Can you work these out from the model? Positions are in its coordinate system, mm. A direction names the side the tool comes from. Coordinates: 2 decimals unless noted, no trailing zeros. Order: outer loops, then holes, each group sorted by start corner. A loop starts at its lowest first (then second) coordinate and runs counter-clockwise, first axis right, second up.
```python
from build123d import *

# Parameters (mm, degrees)
EXTRUDE_1_DEPTH     = 10
SKETCH_2_R          = 1.25
CUT_EXTRUDE_1_DEPTH = 15
SKETCH_4_R          = 0.95
CUT_EXTRUDE_2_DEPTH = 40.749213829
EXTRUDE_2_DEPTH     = 28
SKETCH_7_W          = 6
SKETCH_7_H          = 20
EXTRUDE_4_DEPTH     = 2
CHAMFER_1_SIZE      = 0.6
EXTRUDE_5_DEPTH     = 10
FILLET_2_R          = 6
CUT_EXTRUDE_3_DEPTH = 1
CHAMFER_2_SIZE      = 1


# Some blends are built 0.0001 mm under size
with BuildPart() as part:
    # 草图1 → 凸台-拉伸1 (new, symmetric)
    with BuildSketch(Plane(origin=(0, 0, 0), x_dir=(1, 0, 0), z_dir=(0, 1, 0))):
        Polygon((0, 0), (3, 0), (3, 10), (1, 10), (1, 2), (-2, 2), (-2, -26), (-6, -26), (-6, -28), (0, -28), align=None)
    extrude(amount=EXTRUDE_1_DEPTH, both=True)

    # 草图2 → 切除-拉伸1 (cut)
    with BuildSketch(Plane.ZY.offset(-1)):
        with Locations((-5, 0)):
            Circle(SKETCH_2_R)
    extrude(amount=-CUT_EXTRUDE_1_DEPTH, mode=Mode.SUBTRACT)

    # 草图4 → 切除-拉伸2 (cut, through all)
    with BuildSketch(Plane.XY.offset(28)):
        with Locations((-4, 0)):
            Circle(SKETCH_4_R)
    extrude(amount=-CUT_EXTRUDE_2_DEPTH, mode=Mode.SUBTRACT)

    # 草图5 → 凸台-拉伸2 (add)
    with BuildSketch(Plane(origin=(0, 0, 26), x_dir=(-1, 0, 0), z_dir=(0, 0, -1))):
        Polygon((2, 10), (6, 10), (2, 6), align=None)
        Polygon((2, -6), (2, -10), (6, -10), align=None)
    extrude(amount=EXTRUDE_2_DEPTH)

    # 草图7 → 凸台-拉伸4 (add)
    with BuildSketch(Plane(origin=(0, 0, -10), x_dir=(-1, 0, 0), z_dir=(0, 0, -1))):
        with Locations((-4, 0)):
            Rectangle(SKETCH_7_W, SKETCH_7_H)
    extrude(amount=EXTRUDE_4_DEPTH)

    # 倒角1
    chamfer_1_edges = [part.edges().sort_by_distance(p)[0] for p in [
        (5, 10, -10),
        (5, -10, -10),
    ]]
    chamfer(chamfer_1_edges, length=CHAMFER_1_SIZE)

    # 草图8 → 凸台-拉伸5 (add)
    with BuildSketch(Plane(origin=(0, 0, -2), x_dir=(-1, 0, 0), z_dir=(0, 0, -1))):
        Polygon((-1, 10), (1.5, 10), (-1, 7.5), align=None)
        Polygon((-1, -7.5), (-1, -10), (1.5, -10), align=None)
    extrude(amount=EXTRUDE_5_DEPTH)

    # 圆角2
    # the kernel refuses this fillet: 6 mm, written as the material it adds along each edge
    with BuildSketch(Plane(origin=(-12.106601718, -20.606601718, -2), x_dir=(-0.7071067811865437, 0.7071067811865513, 0), z_dir=(0.7071067811865513, 0.7071067811865438, 0))) as fillet_2_piece_1_section:
        with BuildLine():
            CenterArc((FILLET_2_R, -FILLET_2_R), FILLET_2_R, 90, 90)
            Line((0, -FILLET_2_R), (0, 0))
            Line((0, 0), (FILLET_2_R, 0))
        make_face()
    fillet_2_piece_1 = extrude(amount=33.535533906, mode=Mode.PRIVATE)
    fillet_2_piece_1 = split(fillet_2_piece_1, bisect_by=Plane(origin=(-2, -8.855149606, -2.774001208), z_dir=(-1, 0, 0)), keep=Keep.TOP, mode=Mode.PRIVATE)
    fillet_2_piece_1 = split(fillet_2_piece_1, bisect_by=Plane(origin=(-4, -8, -2.774001208), z_dir=(0.7071067811865515, -0.7071067811865436, 0)), keep=Keep.TOP, mode=Mode.PRIVATE)
    fillet_2_piece_1 = split(fillet_2_piece_1, bisect_by=Plane(origin=(-3.144850394, -10, -2.774001208), z_dir=(0, 1, 0)), keep=Keep.TOP, mode=Mode.PRIVATE)
    add(fillet_2_piece_1)
    with BuildSketch(Plane(origin=(-12.106601718, -20.606601718, -2), x_dir=(-0.7071067811865437, 0.7071067811865513, 0), z_dir=(0.7071067811865513, 0.7071067811865438, 0))) as fillet_2_piece_2_section:
        with BuildLine():
            CenterArc((FILLET_2_R, -FILLET_2_R), FILLET_2_R, 90, 90)
            Line((0, -FILLET_2_R), (0, 0))
            Line((0, 0), (FILLET_2_R, 0))
        make_face()
    fillet_2_piece_2 = extrude(amount=33.535533906, mode=Mode.PRIVATE)
    fillet_2_piece_2 = split(fillet_2_piece_2, bisect_by=Plane(origin=(1, -3.168547951, -2.116110368), z_dir=(-1, 0, 0)), keep=Keep.TOP, mode=Mode.PRIVATE)
    fillet_2_piece_2 = split(fillet_2_piece_2, bisect_by=Plane(origin=(-2, -3.168547951, -2.116110368), z_dir=(1, 0, 0)), keep=Keep.TOP, mode=Mode.PRIVATE)
    fillet_2_piece_2 = split(fillet_2_piece_2, bisect_by=Plane(origin=(0.165726024, -3.834273976, -2.116110368), z_dir=(-0.7071067811865515, 0.7071067811865436, 0)), keep=Keep.TOP, mode=Mode.PRIVATE)
    add(fillet_2_piece_2)
    with BuildSketch(Plane(origin=(-12.106601718, -20.606601718, -2), x_dir=(-0.7071067811865437, 0.7071067811865513, 0), z_dir=(0.7071067811865513, 0.7071067811865438, 0))) as fillet_2_piece_3_section:
        with BuildLine():
            CenterArc((FILLET_2_R, -FILLET_2_R), FILLET_2_R, 90, 90)
            Line((0, -FILLET_2_R), (0, 0))
            Line((0, 0), (FILLET_2_R, 0))
        make_face()
    fillet_2_piece_3 = extrude(amount=33.535533906, mode=Mode.PRIVATE)
    fillet_2_piece_3 = split(fillet_2_piece_3, bisect_by=Plane(origin=(1, -7.448559775, -3.464262476), z_dir=(-1, 0, 0)), keep=Keep.TOP, mode=Mode.PRIVATE)
    fillet_2_piece_3 = split(fillet_2_piece_3, bisect_by=Plane(origin=(-2, -7.448559775, -3.464262476), z_dir=(1, 0, 0)), keep=Keep.TOP, mode=Mode.PRIVATE)
    fillet_2_piece_3 = split(fillet_2_piece_3, bisect_by=Plane(origin=(-1.950921276, -5.950921276, -3.464262476), z_dir=(0.7071067811865515, -0.7071067811865436, 0)), keep=Keep.TOP, mode=Mode.PRIVATE)
    fillet_2_piece_3 = split(fillet_2_piece_3, bisect_by=Plane(origin=(-0.453282777, -10, -3.464262476), z_dir=(0, 1, 0)), keep=Keep.TOP, mode=Mode.PRIVATE)
    add(fillet_2_piece_3)
    with BuildSketch(Plane(origin=(-12.106601718, 20.606601718, -2), x_dir=(-0.707106781186544, -0.7071067811865511, 0), z_dir=(0.7071067811865511, -0.7071067811865439, 0))) as fillet_2_piece_4_section:
        with BuildLine():
            CenterArc((FILLET_2_R, FILLET_2_R), FILLET_2_R, 180, 90)
            Line((0, FILLET_2_R), (0, 0))
            Line((0, 0), (FILLET_2_R, 0))
        make_face()
    fillet_2_piece_4 = extrude(amount=33.535533906, mode=Mode.PRIVATE)
    fillet_2_piece_4 = split(fillet_2_piece_4, bisect_by=Plane(origin=(-3.144850394, 10, -2.774001208), z_dir=(0, -1, 0)), keep=Keep.TOP, mode=Mode.PRIVATE)
    fillet_2_piece_4 = split(fillet_2_piece_4, bisect_by=Plane(origin=(-4, 8, -2.774001208), z_dir=(0.7071067811865515, 0.7071067811865436, 0)), keep=Keep.TOP, mode=Mode.PRIVATE)
    fillet_2_piece_4 = split(fillet_2_piece_4, bisect_by=Plane(origin=(-2, 8.855149606, -2.774001208), z_dir=(-1, 0, 0)), keep=Keep.TOP, mode=Mode.PRIVATE)
    add(fillet_2_piece_4)
    with BuildSketch(Plane(origin=(-12.106601718, 20.606601718, -2), x_dir=(-0.707106781186544, -0.7071067811865511, 0), z_dir=(0.7071067811865511, -0.7071067811865439, 0))) as fillet_2_piece_5_section:
        with BuildLine():
            CenterArc((FILLET_2_R, FILLET_2_R), FILLET_2_R, 180, 90)
            Line((0, FILLET_2_R), (0, 0))
            Line((0, 0), (FILLET_2_R, 0))
        make_face()
    fillet_2_piece_5 = extrude(amount=33.535533906, mode=Mode.PRIVATE)
    fillet_2_piece_5 = split(fillet_2_piece_5, bisect_by=Plane(origin=(1, 3.168547951, -2.116110368), z_dir=(-1, 0, 0)), keep=Keep.TOP, mode=Mode.PRIVATE)
    fillet_2_piece_5 = split(fillet_2_piece_5, bisect_by=Plane(origin=(0.165726024, 3.834273976, -2.116110368), z_dir=(-0.7071067811865515, -0.7071067811865436, 0)), keep=Keep.TOP, mode=Mode.PRIVATE)
    fillet_2_piece_5 = split(fillet_2_piece_5, bisect_by=Plane(origin=(-2, 3.168547951, -2.116110368), z_dir=(1, 0, 0)), keep=Keep.TOP, mode=Mode.PRIVATE)
    add(fillet_2_piece_5)
    with BuildSketch(Plane(origin=(-12.106601718, 20.606601718, -2), x_dir=(-0.707106781186544, -0.7071067811865511, 0), z_dir=(0.7071067811865511, -0.7071067811865439, 0))) as fillet_2_piece_6_section:
        with BuildLine():
            CenterArc((FILLET_2_R, FILLET_2_R), FILLET_2_R, 180, 90)
            Line((0, FILLET_2_R), (0, 0))
            Line((0, 0), (FILLET_2_R, 0))
        make_face()
    fillet_2_piece_6 = extrude(amount=33.535533906, mode=Mode.PRIVATE)
    fillet_2_piece_6 = split(fillet_2_piece_6, bisect_by=Plane(origin=(1, 7.448559775, -3.464262476), z_dir=(-1, 0, 0)), keep=Keep.TOP, mode=Mode.PRIVATE)
    fillet_2_piece_6 = split(fillet_2_piece_6, bisect_by=Plane(origin=(-0.453282777, 10, -3.464262476), z_dir=(0, -1, 0)), keep=Keep.TOP, mode=Mode.PRIVATE)
    fillet_2_piece_6 = split(fillet_2_piece_6, bisect_by=Plane(origin=(-1.950921276, 5.950921276, -3.464262476), z_dir=(0.7071067811865515, 0.7071067811865436, 0)), keep=Keep.TOP, mode=Mode.PRIVATE)
    fillet_2_piece_6 = split(fillet_2_piece_6, bisect_by=Plane(origin=(-2, 7.448559775, -3.464262476), z_dir=(1, 0, 0)), keep=Keep.TOP, mode=Mode.PRIVATE)
    add(fillet_2_piece_6)

    # 草图9 → 切除-拉伸3 (cut)
    with BuildSketch(Plane(origin=(3, 0, 0), x_dir=(0, 0, -1), z_dir=(1, 0, 0))):
        with BuildLine():
            Line((0, -3), (0, 3))
            Line((0, 3), (5.378333925, 1.963889875))
            ThreePointArc((5.378333925, 1.963889875), (7, 0), (5.378333925, -1.963889875))
            Line((5.378333925, -1.963889875), (0, -3))
        make_face()
    extrude(amount=-CUT_EXTRUDE_3_DEPTH, mode=Mode.SUBTRACT)

    # 倒角2
    chamfer_2_edges = [part.edges().sort_by_distance(p)[0] for p in [
        (3, -2.481944938, -2.689166963),
        (3, 0, -7),
        (3, 2.481944938, -2.689166963),
    ]]
    chamfer(chamfer_2_edges, length=CHAMFER_2_SIZE - 0.0001)  # a hair under: the kernel refuses the full size


solid = part.part
```
1. Thinking about a two-plate mould opening in Y: for faces 4 (the flat face through (0, 0, 14)), 5 (the flat face through (2.49, 2.99, -2.65)), 6 (the flat face through (-2, -10, 8)), 7 (the flat face through (-0.3, -8.8, -10)), which applies, pulls with the +Y half, pulls with the -Y half, needs draft (parallel to the pull), parting line crosses it, or undercut?
Completed:
face 4: needs draft
face 5: undercut
face 6: pulls with the -Y half
face 7: undercut
2. Please list where these lines run through material, in increasing order: probe 1 along Y at (x, z) = (1.45, -5); probe 2 along Y at (x, z) = (-3.5, 22); probe 3 along Z at (x, y) = (-4, 4.5).
Completed:
probe 1: y = -10 to -1.25, 1.25 to 10
probe 2: y = -10 to -7.5, 7.5 to 10
probe 3: z = 26 to 28
3. Imagine slicing it at B-B on z = 5.5. Please give me the cut outline in (x, y), then the cut area to 3 significant figures.
Completed:
outline: (-6, -10) - (0, -10) - (0, 10) - (-6, 10) - (-2, 6) - (-2, -6) - close
area: 56.0 mm2
4. I'm going to push flat-ended pins straight in: pin 1 (1 mm diameter, centred on x = -1, y = -0.5, fed in from -Z); pin 2 (5 mm diameter, centred on y = -6.5, z = 4, fed in from +X); pin 3 (11.5 mm diameter, centred on y = -2, z = -5.5, fed in from +X); pin 4 (2 mm diameter, centred on x = -5, y = -3, fed in from -Z). Where does each tip first touch, or does it pass through?
Completed:
pin 1: stops at z = -2
pin 2: stops at x = 0
pin 3: stops at x = 7
pin 4: stops at z = 26
5. On a 3-axis mill with a long thin cutter (end or side, diameter ignored), from which of +Z, -Z, +X, -X, +Y, -Y can I reach the whole of each face in a straight line? I mean faces 1 (the conical face through (2.2, 0, -7.2)), 2 (the flat face through (-4, -8, 12)), 3 (the flat face through (1, 0, 0)). Say none if no direction works.
Completed:
face 1: +Z, +X
face 2: -Z, -X
face 3: +Z, +X, +Y, -Y
